Autodesk Inventor part; units mm, degrees
ref_plane "YZ Plane" through (0, 0, 0) normal (1, 0, 0) x (0, 1, 0)
ref_plane "XZ Plane" through (0, 0, 0) normal (0, 1, 0) x (-1, 0, 0)
ref_plane "XY Plane" through (0, 0, 0) normal (0, 0, 1) x (1, 0, 0)
ref_plane "Work Plane1" through (13.7597, -5.7182, -8.0415) normal (0, -1, 0) x (1, 0, 0)
sketch "Sketch1" plane through (13.7597, -5.7182, -8.0415) normal (0, -1, 0) x (1, 0, 0)
  line L0 (8.0899, -8.0899) -> (8.0899, 8.0899) construction
  line L1 (8.0899, 8.0899) -> (-8.0899, 8.0899) construction
  line L2 (-8.0899, 8.0899) -> (-8.0899, -8.0899) construction
  line L3 (-8.0899, -8.0899) -> (8.0899, -8.0899) construction
  line L4 (8.0899, 8.0899) -> (-15.7007, 8.0899)
  line L5 (-15.7007, 8.0899) -> (-15.7007, 9.3894)
  line L6 (-15.7007, 9.3894) -> (8.0899, 9.3894)
  line L7 (8.0899, 9.3894) -> (8.0899, 8.0899)
  line L8 (8.0899, -8.0899) -> (-15.7007, -8.0899)
  line L9 (-15.7007, -8.0899) -> (-15.7007, -9.3894)
  line L10 (-15.7007, -9.3894) -> (8.0899, -9.3894)
  line L11 (8.0899, -9.3894) -> (8.0899, -8.0899)
  point P0 (-13.7597, 8.0415)
extrude "Extrusion1" add sketch "Sketch1" against normal blind 17.4625
sketch "Sketch2" plane through (21.8496, -5.7182, -17.4309) normal (0, 0, -1) x (-1, 0, 0)
  circle A0 centre (11.8953, 8.705) radius 1.7859
  line L0 (23.6468, 17.41) -> (0, 0) construction
  line L1 (0, 0) -> (23.7906, 0) construction
  line L2 (23.7906, 0) -> (0, 17.41) construction
  point P0 (21.8496, 5.7182)
extrude "Extrusion2" cut sketch "Sketch2" against normal through all
sketch "Sketch3" plane through (13.7597, 11.7443, -8.0415) normal (0, 1, 0) x (1, 0, 0)
  line L0 (-15.7007, -9.3894) -> (8.0899, -9.3894) construction
  line L1 (-15.7007, -8.0899) -> (-15.7007, -9.3894) construction
  line L2 (8.0899, 9.3894) -> (-15.7007, 9.3894) construction
  line L3 (8.0899, 8.0899) -> (8.0899, 9.3894) construction
  line L4 (-15.7007, -9.3894) -> (8.0899, -9.3894)
  line L5 (8.0899, -9.3894) -> (8.0899, 9.3894)
  line L6 (8.0899, 9.3894) -> (-15.7007, 9.3894)
  line L7 (-15.7007, 9.3894) -> (-15.7007, -9.3894)
  point P0 (-13.7597, -8.0415)
extrude "Extrusion3" add sketch "Sketch3" along normal blind 1.5875
sketch "Sketch5" plane through (13.7597, 11.7443, -8.0415) normal (0, -1, 0) x (1, 0, 0)
  point P0 (-13.7597, 8.0415)
sketch "Sketch6" plane through (13.7597, 11.7443, -8.0415) normal (0, -1, 0) x (1, 0, 0)
  circle A0 centre (-4.1928, -0.2672) radius 4
  point P0 (-13.7597, 8.0415)
extrude "Extrusion5" cut sketch "Sketch6" against normal through all
Read the model definition and answer for the solid it produces. Units are mm, in the model's axes. A direction names the side the tool comes from. Coordinates: 2 decimals unless noted, no trailing zeros. Loops run counter-clockwise (first coordinate to the right, second up) from the corner with the lowest first, then second, coordinate; pieces in that order, holes last. Notation, with made-up numbers: (60.5, 5.5) -> (110.5, 5.5) arc R31 cw to (110.5, 44.5) -> close; hole circle Ø6 at (-17.5, 7.5). An arc over 180 degrees is marked (long way). Answer in a Markdown table with one row per item.
Item 1: For faces 1 (the flat face through (10, 1, -16.131)), 2 (the flat face through (-1.941, 12, -8)), determine the directions among +Z, -Z, +X, -X, +Y, -Y from which every point of the face is accessible in a straight line to the end or side of a thin tool.
Returned:
| item | result |
|---|---|
| face 1 | +X, -X, -Y |
| face 2 | +Z, -Z, -X, +Y, -Y |
Item 2: A cutting plane is placed at D-D on y = 4. Determine the outline of the cut face in (x, z).
Returned:
| item | result |
|---|---|
| outline | (-1.94, -17.43) -> (8.48, -17.43) -> (8.48, -16.13) -> (-1.94, -16.13) -> close; (-1.94, 0.05) -> (8.48, 0.05) -> (8.48, 1.35) -> (-1.94, 1.35) -> close; (11.42, -17.43) -> (21.85, -17.43) -> (21.85, -16.13) -> (11.42, -16.13) -> close; (11.42, 0.05) -> (21.85, 0.05) -> (21.85, 1.35) -> (11.42, 1.35) -> close |
Item 3: A cutting plane is placed at B-B on x = 13. Determine the outline of the cut face in (y, z), plus the area to 3 significant figures.
Returned:
| item | result |
|---|---|
| outline | (-5.72, -17.43) -> (13.33, -17.43) -> (13.33, -10.36) -> (11.74, -10.36) -> (11.74, -16.13) -> (-5.72, -16.13) -> close; (-5.72, 0.05) -> (11.74, 0.05) -> (11.74, -6.26) -> (13.33, -6.26) -> (13.33, 1.35) -> (-5.72, 1.35) -> close |
| area | 68.7 mm^2 |
Item 4: A cutting plane is placed at C-C on z = -9.5. Determine the outline of the cut face in (x, y).
Returned:
| item | result |
|---|---|
| outline | (-1.94, 11.74) -> (5.75, 11.74) -> (5.75, 13.33) -> (-1.94, 13.33) -> close; (13.39, 11.74) -> (21.85, 11.74) -> (21.85, 13.33) -> (13.39, 13.33) -> close |
Item 5: Straight lines are drawn through the part: line 1 along Z through (x, y) = (15.5, -2.25); line 2 along Y through (x, z) = (16.75, -13.75). For each, find the intervals that lie inside material, in ascending order. Write a range as [from, to].
Returned:
| item | result |
|---|---|
| line 1 | z = [-17.43, -16.13], [0.05, 1.35] |
| line 2 | y = [11.74, 13.33] |
Item 6: This flat-tipped pin is pushed along its axis until it touches: P1, Ø8, axis at x = 10.5, z = -6, coming from the -Y side. Where does it stop, or does it pass through?
Returned:
| item | result |
|---|---|
| P1 | stops at y = 11.74 |
Item 7: A cutting plane is placed at A-A on y = -2.5. Determine the outline of the cut face in (x, z), plus the area to 3 significant figures.
Returned:
| item | result |
|---|---|
| outline | (-1.94, -17.43) -> (21.85, -17.43) -> (21.85, -16.13) -> (-1.94, -16.13) -> close; (-1.94, 0.05) -> (21.85, 0.05) -> (21.85, 1.35) -> (-1.94, 1.35) -> close |
| area | 61.8 mm^2 |
Item 8: For a pull along X with two mould halves and no side action, classify faces 3 (the flat face through (21.85, 12, -8)), 4 (the flat face through (10, 6, -17.431)), 5 (the cylindrical face through (11.74, 3.07, -16.79)) as released by +X, released by -X, zero draft, split by the parting line, or undercut.
Returned:
| item | result |
|---|---|
| face 3 | released by +X |
| face 4 | zero draft |
| face 5 | undercut |
